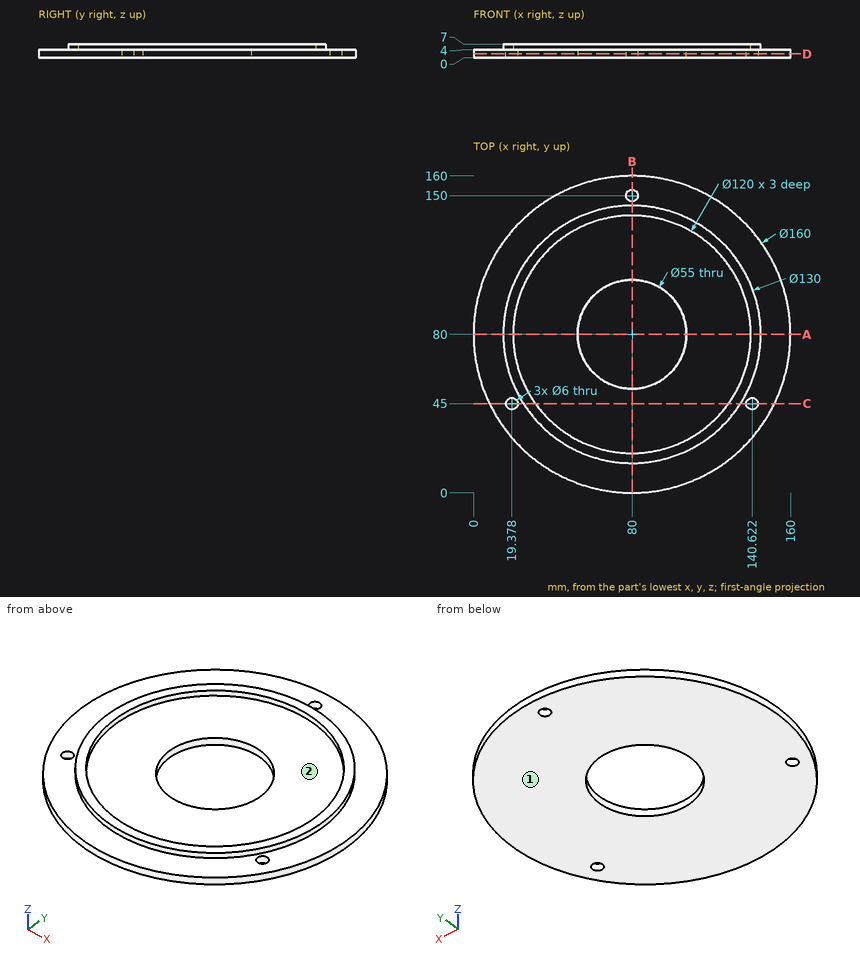
Print and shaded views of the part. All mm, measured from the part's lowest x, y and z. Coordinates: 2 decimals unless noted, no trailing zeros. Write each loop counter-clockwise with the first axis right and the second up, starting at its lowest first coordinate (ties: lowest second). Pieces come first, ordered by that corner, then holes. Notation, with made-up numbers: (8, 82) - (16, 82) arc R31 cw to (16, 114) - close; hole circle Ø1 at (71.5, -7). An arc over 180 degrees is marked (long way). One line per question, with ' | ' between items. Start each with the question number.
Q1. Cut at B-B, the plane x = 80. List the corners of the cut face in (y, z).
Q2. Cut at D-D, the plane z = 2. List the corners of the cut face in (x, y), then the cut area to 3 significant figures.
Q3. Pull direction X, two halves, no side cores. Call the marked faces 1 and 2: pulls with the +X half, pulls with the -X half, needs draft (parallel to the pull), parting line crosses it, or undercut.
Q4. Pin check, flat tips, straight feed: pin 1 (1 mm diameter, centred on x = 97.5, y = 102.5, fed in from +Z); pin 2 (12 mm diameter, centred on x = 95.5, y = 70, fed in from -Z); pin 3 (3 mm diameter, centred on y = 112, z = 5, fed in from +X); pin 4 (4 mm diameter, centred on x = 28.5, z = 2.5, fed in from +Y). Stop position of each tip, or through.
Q5. Drill centre lines: line 1 (Y direction, x = 80, z = 1.7); line 2 (Y direction, x = 80, z = 5.65); line 3 (Z direction, x = 45, y = 102). Where is each one in solid material? Low to high. Write a range as [from, to].
Q6. Cut at A-A, the plane y = 80. List the corners of the cut face in (x, z).
Q7. Cut at C-C, the plane y = 45. List the corners of the cut face in (x, z), then the cut area to 3 significant figures.
Answer below:
1) outline: (0, 0) - (52.5, 0) - (52.5, 4) - (20, 4) - (20, 7) - (15, 7) - (15, 4) - (0, 4) - close; (107.5, 0) - (147, 0) - (147, 4) - (145, 4) - (145, 7) - (140, 7) - (140, 4) - (107.5, 4) - close; (153, 0) - (160, 0) - (160, 4) - (153, 4) - close
2) outline: circle Ø160 at (80, 80); hole circle Ø6 at (19.38, 45); hole circle Ø55 at (80, 80); hole circle Ø6 at (80, 150); hole circle Ø6 at (140.62, 45) | area: 17,600 mm^2
3) face 1: needs draft | face 2: undercut
4) pin 1: z = 4 | pin 2: through | pin 3: x = 153.8 | pin 4: y = 142.85
5) line 1: [0, 52.5], [107.5, 147], [153, 160] | line 2: [15, 20], [140, 145] | line 3: [0, 4]
6) outline: (0, 0) - (52.5, 0) - (52.5, 4) - (20, 4) - (20, 7) - (15, 7) - (15, 4) - (0, 4) - close; (107.5, 0) - (160, 0) - (160, 4) - (145, 4) - (145, 7) - (140, 7) - (140, 4) - (107.5, 4) - close
7) outline: (8.06, 0) - (16.38, 0) - (16.38, 4) - (8.06, 4) - close; (22.38, 0) - (137.62, 0) - (137.62, 4) - (134.77, 4) - (134.77, 7) - (128.73, 7) - (128.73, 4) - (31.27, 4) - (31.27, 7) - (25.23, 7) - (25.23, 4) - (22.38, 4) - close; (143.62, 0) - (151.94, 0) - (151.94, 4) - (143.62, 4) - close | area: 564 mm^2
